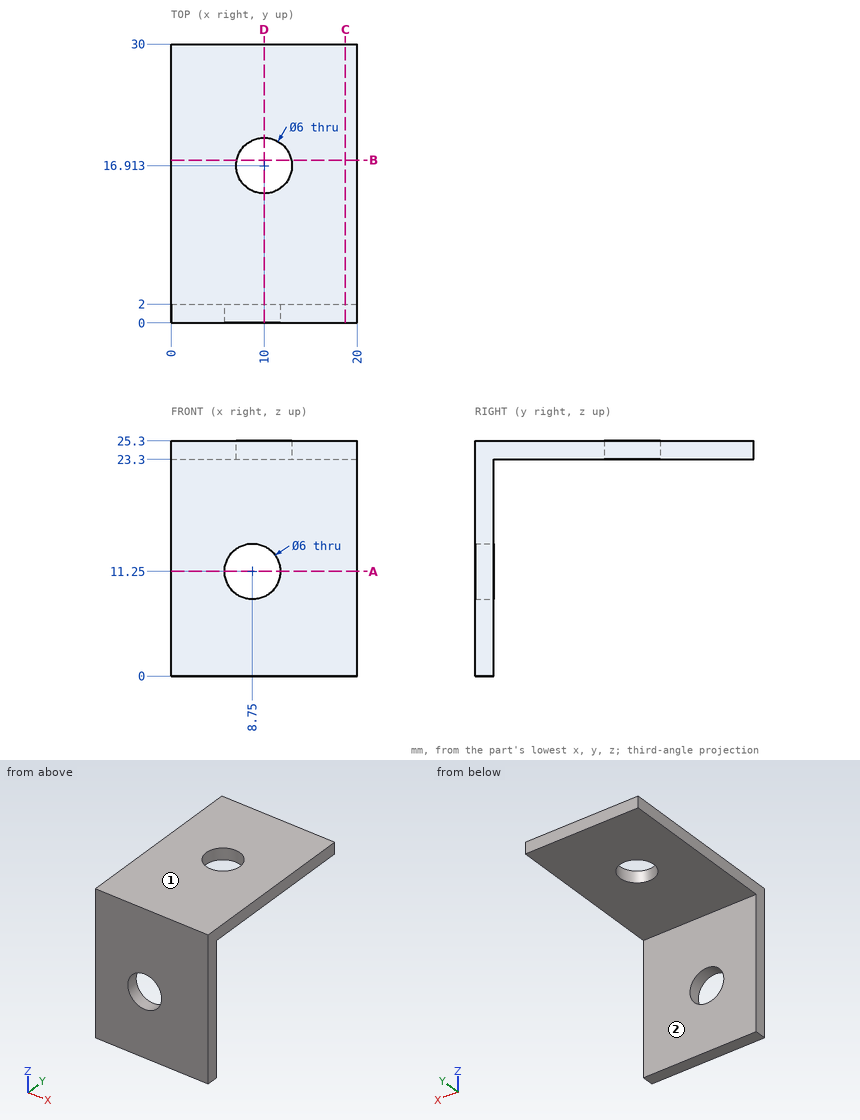
Design review of the part shown in the three views and the two pictorial views. Dimensions are in mm from the part's minimum x, y and z. A direction names the side the tool comes from. Round coordinates to 2 decimals unless told otherwise and drop trailing zeros. Write each loop counter-clockwise with the first axis right and the second up, starting at its lowest first coordinate (ties: lowest second). Pieces come first, ordered by that corner, then holes.
1) Take a section at C-C on x = 18.75. Give the boundary of the cut face in (y, z), then the cut area to 3 significant figures.
Answer below:
outline: (0, 0) - (2, 0) - (2, 23.3) - (30, 23.3) - (30, 25.3) - (0, 25.3) - close
area: 107 mm2
2) Insertion check: pin 1 Ø2 at (x, y) = (14, 10.5) entering from -Z; pin 2 Ø2 at (x, y) = (10, 16) entering from -Z; pin 3 Ø9.5 at (x, z) = (8.75, 11.25) entering from +Y. Each pin has a flat end and moves straight along its axis. Give the tip position at first contact, or say it passes through.
Answer below:
pin 1: stops at z = 23.3
pin 2: passes through
pin 3: stops at y = 2
3) Take a section at B-B on y = 17.5. Give the boundary of the cut face in (x, z), then the cut area to 3 significant figures.
Answer below:
outline: (0, 23.3) - (7.06, 23.3) - (7.06, 25.3) - (0, 25.3) - close; (12.94, 23.3) - (20, 23.3) - (20, 25.3) - (12.94, 25.3) - close
area: 28.2 mm2
4) Machinability: for the marked faces 1 and 2, which of the approach directions +Z, -Z, +X, -X, +Y, -Y give a long, thin tool a straight path to every point of the face, cutting with its end or side? Answer none if there is none.
Answer below:
face 1: +Z, +X, -X, +Y, -Y
face 2: -Z, +X, -X, +Y
5) For line 1 along X through (y, z) = (0.6, 11.25); line 2 along Y through (x, z) = (10, 24.95); line 3 along Z through (x, y) = (8, 21.25), list the stretches that pass through material, from the lowest coordinate up.
Answer below:
line 1: x = 0 to 5.75, 11.75 to 20
line 2: y = 0 to 13.91, 19.91 to 30
line 3: z = 23.3 to 25.3
6) Take a section at D-D on x = 10. Give the boundary of the cut face in (y, z).
Answer below:
outline: (0, 0) - (2, 0) - (2, 8.52) - (0, 8.52) - close; (0, 13.98) - (2, 13.98) - (2, 23.3) - (13.91, 23.3) - (13.91, 25.3) - (0, 25.3) - close; (19.91, 23.3) - (30, 23.3) - (30, 25.3) - (19.91, 25.3) - close
7) Take a section at A-A on z = 11.25. Give the boundary of the cut face in (x, y), then the cut area to 3 significant figures.
Answer below:
outline: (0, 0) - (5.75, 0) - (5.75, 2) - (0, 2) - close; (11.75, 0) - (20, 0) - (20, 2) - (11.75, 2) - close
area: 28.0 mm2
